For this review, take the finished solid that the model builds, in its own axes (mm). A direction names the side the tool comes from. Round coordinates to 2 decimals unless told otherwise and drop trailing zeros. Order: outer loops, then holes, each group sorted by start corner. A loop starts at its lowest first (then second) coordinate and runs counter-clockwise, first axis right, second up. Notation, with made-up numbers: M -18,52.25 L 16,52.25 A17 cw 16,71.25 Z; hole C -39.5,67.25 d8. An arc over 180 degrees is marked long. Answer as a JSON object with one key per item and string values.
from build123d import *


with BuildPart() as part:
    # Sketch1 → Revolve1 (revolve)
    with BuildSketch(Plane.XY):
        Polygon((0, 0), (0, 6.50875), (0.762, 7.27075), (2.7178, 7.27075), (3.3528, 6.63575), (3.9878, 6.63575), (3.9878, 7.8105), (12.7508, 7.8105), (13.5128, 7.0485), (13.5128, 0), align=None)
    revolve(axis=Axis((13.5128, 0, 0), (-1, 0, 0)))

    # Sketch2 → Cut-Revolve1 (revolve, cut)
    with BuildSketch(Plane.XY):
        Polygon((0, 0), (0, 1.9558), (12.2936, 1.9558), (13.422781656, 0), align=None)
    revolve(axis=Axis((13.422781656, 0, 0), (-1, 0, 0)), mode=Mode.SUBTRACT)

    # Sketch3 → Cut-Revolve2 (revolve, cut)
    with BuildSketch(Plane(origin=(0, 0, 0), x_dir=(1, 0, 0), z_dir=(0, 1, 0))):
        Polygon((10.3124, 0), (12.29614, 0), (12.29614, -6.36524), (12.7254, -6.7945), (14.2748, -6.7945), (14.2748, -7.8105), (10.3124, -7.8105), align=None)
    revolve(axis=Axis((10.3124, 0, 7.8105), (0, 0, -1)), mode=Mode.SUBTRACT)

    # Sketch4 → Revolve2 (revolve)
    with BuildSketch(Plane.XY):
        with BuildLine():
            Line((3.160243808, 7.8105), (3.160243808, 7.726331804))
            Line((3.160243808, 7.726331804), (3.870760245, 7.015815367))
            ThreePointArc((3.870760245, 7.015815367), (3.907957684, 6.926012806), (3.870760245, 6.836210245))
            Line((3.870760245, 6.836210245), (3.6703, 6.63575))
            Line((3.6703, 6.63575), (3.3528, 6.63575))
            Line((3.3528, 6.63575), (3.3528, 6.38175))
            Line((3.3528, 6.38175), (3.9878, 6.38175))
            Line((3.9878, 6.38175), (3.9878, 7.186143808))
            Line((3.9878, 7.186143808), (3.363443808, 7.8105))
            Line((3.363443808, 7.8105), (3.160243808, 7.8105))
        make_face()
    revolve(axis=Axis((3.9878, 0, 0), (-1, 0, 0)))


solid = part.part
1) Add section C-C on x = 2. State the section outline as (y, z) points, and give its area (3 significant figures).
Geometry check:
{"outline": "C 0,0 d14.54; hole C 0,0 d3.91", "area": "154 mm²"}
2) For L1, parallel to X at y = 0, z = 3.75; L2, parallel to Y at x = 7.25, z = 0; L3, parallel to Z at x = 2.5, y = 0, list the stretches that pass through material, from the lowest coordinate up.
Geometry check:
{"L1": "x = 0 to 8.33, 12.3 to 13.51", "L2": "y = -7.81 to -1.96, 1.96 to 7.81", "L3": "z = -7.27 to -1.96, 1.96 to 7.27"}
3) Insertion check: P1, Ø1, axis at x = 3.5, y = -5, coming from the +Z side; P2, Ø2, axis at x = 11, y = 1, coming from the +Z side; P3, Ø6.5, axis at x = 10.31, y = 0, coming from the +Z side. Each pin has a flat end and moves straight along its axis. Give the tip position at first contact, or say it passes through.
Geometry check:
{"P1": "stops at z = 6.37", "P2": "stops at z = 6.6", "P3": "stops at z = 6.79"}
4) Mouldability with a two-part tool opening along X and no side actions: class faces 4 (the flat face through (13.513, -0.1, -0.2)), 5 (the flat face through (0, -1, -2)), 6 (the cylindrical face through (11.23, 1.76, 3.93)) as +X half, -X half, draft (parallel to the pull), parting line (faces both ways), or undercut.
Geometry check:
{"face 4": "+X half", "face 5": "-X half", "face 6": "undercut"}
5) Machinability: for faces 1 (the cylindrical face through (6.35, -0.07, 7.2)), 2 (the cylindrical face through (1.75, -5.36, -4.91)), 3 (the cylindrical face through (3.51, 3.06, 5.89)), which of the approach directions +Z, -Z, +X, -X, +Y, -Y give a long, thin tool a straight path to every point of the face, cutting with its end or side? Answer none if there is none.
Geometry check:
{"face 1": "+Z", "face 2": "-X", "face 3": "none"}
6) Add section B-B on x = 7.5. State the section outline as (y, z) points.
Geometry check:
{"outline": "M -2.79,6.79 L -2.79,7.29 A7.81 ccw long 2.79,7.29 L 2.79,6.79 Z; hole C 0,0 d3.91"}
7) Add section A-A on x = 5.25. State the section outline as (y, z) points.
Geometry check:
{"outline": "C 0,0 d15.62; hole C 0,0 d3.91"}
